Check sheet for the modelled part. Datum: model origin and axes. Units: mm. A direction names the side the tool comes from. Round coordinates to 2 decimals unless told otherwise and drop trailing zeros. Loops run counter-clockwise (first coordinate to the right, second up) from the corner with the lowest first, then second, coordinate; pieces in that order, holes last. Notation, with made-up numbers: (65.5, 0.25) - (118.5, 0.25) arc R18 cw to (118.5, 33.25) - close; hole circle Ø9 at (87.5, -2). An arc over 180 degrees is marked (long way). Put each result on its own line as item: value. Start each with the question number.
Item 1: Gauge pin test, flat ends, axial feed: pin 1 Ø2.5 at (x, z) = (75, -18.75) entering from +Y; pin 2 Ø1 at (x, y) = (-58, 1) entering from -Z. Record the tip position at first contact, or that the pin passes through.
Item 2: Section check B-B, the plane z = 48. Record the cut outline in (x, y), and give its area (3 significant figures).
Item 3: Material ranges on line 1 along X through (y, z) = (2.55, -18.75); line 2 along Z through (x, y) = (60, 1.9); line 3 along X through (y, z) = (1.1, 41), recorded low to high.
Item 4: Section check C-C, the plane x = 47.5. Record the cut outline in (y, z).
Item 5: Section check A-A, the plane y = 1.55. Give the number of separate pieces and of enclosed holes in the cut face, and give its area (3 significant figures).
Item 6: Tool access check on faces 1 (the flat face through (68.25, 2, 54)), 2 (the flat face through (-53, 2, -35.75)), 3 (the flat face through (53, 2, -35.75)), 4 (the flat face through (-68.25, 2, 54)), 5 (the flat face through (1, 2, 72.25)). Record the directions out of +Z, -Z, +X, -X, +Y, -Y that give a thin tool (end or side, any length) a straight path to the whole face; none if there is none.
from build123d import *

# Parameters (mm, degrees)
SKETCH1_R           = 1.5025
BOSS_EXTRUDE1_DEPTH = 3.25


with BuildPart() as part:
    # Sketch1 → Boss-Extrude1 (new body)
    with BuildSketch(Plane(origin=(0, 0, 0), x_dir=(1, 0, 0), z_dir=(0, 1, 0))):
        Polygon((-11, 56.036176716), (11, 56.036176716), (26, 35.75), (80, 35.75), (80, -35.75), (68.25, -35.75), (68.25, -72.25), (-68.25, -72.25), (-68.25, -35.75), (-80, -35.75), (-80, 35.75), (-26, 35.75), align=None)
        with Locations((-10, 33.75)):
            Circle(SKETCH1_R, mode=Mode.SUBTRACT)
        with Locations((10, 33.75)):
            Circle(SKETCH1_R, mode=Mode.SUBTRACT)
        with Locations((-10, 53.75)):
            Circle(SKETCH1_R, mode=Mode.SUBTRACT)
        with Locations((10, 53.75)):
            Circle(SKETCH1_R, mode=Mode.SUBTRACT)
        with Locations((-25, 23.75)):
            Circle(SKETCH1_R, mode=Mode.SUBTRACT)
        with Locations((25, 23.75)):
            Circle(SKETCH1_R, mode=Mode.SUBTRACT)
        with Locations((-60, 18.75)):
            Circle(SKETCH1_R, mode=Mode.SUBTRACT)
        with Locations((60, 18.75)):
            Circle(SKETCH1_R, mode=Mode.SUBTRACT)
        with Locations((75, 18.75)):
            Circle(SKETCH1_R, mode=Mode.SUBTRACT)
        with Locations((-60, -16.25)):
            Circle(SKETCH1_R, mode=Mode.SUBTRACT)
        with Locations((60, -16.25)):
            Circle(SKETCH1_R, mode=Mode.SUBTRACT)
        with Locations((75, -16.25)):
            Circle(SKETCH1_R, mode=Mode.SUBTRACT)
        with Locations((-25, -41.25)):
            Circle(SKETCH1_R, mode=Mode.SUBTRACT)
        with Locations((25, -41.25)):
            Circle(SKETCH1_R, mode=Mode.SUBTRACT)
        with Locations((-65, -66.25)):
            Circle(SKETCH1_R, mode=Mode.SUBTRACT)
        with Locations((-20, -66.25)):
            Circle(SKETCH1_R, mode=Mode.SUBTRACT)
        with Locations((20, -66.25)):
            Circle(SKETCH1_R, mode=Mode.SUBTRACT)
        with Locations((65, -66.25)):
            Circle(SKETCH1_R, mode=Mode.SUBTRACT)
        with Locations((-75, 18.75)):
            Circle(SKETCH1_R, mode=Mode.SUBTRACT)
        with Locations((-75, -16.25)):
            Circle(SKETCH1_R, mode=Mode.SUBTRACT)
    extrude(amount=BOSS_EXTRUDE1_DEPTH)


solid = part.part
Check result:
1. pin 1: through
1. pin 2: z = -35.75
2. outline: (-68.25, 0) - (68.25, 0) - (68.25, 3.25) - (-68.25, 3.25) - close
2. area: 444 mm²
3. line 1: -80 to -76.5, -73.5 to -61.5, -58.5 to 58.5, 61.5 to 73.5, 76.5 to 80
3. line 2: -35.75 to -20.25, -17.25 to 14.75, 17.75 to 72.25
3. line 3: -68.25 to -26.48, -23.52 to 23.52, 26.48 to 68.25
4. outline: (0, -35.75) - (3.25, -35.75) - (3.25, 72.25) - (0, 72.25) - close
5. separate pieces: 1
5. enclosed holes: 20
5. area: 17,000 mm²
6. face 1: +Z, +X, +Y, -Y
6. face 2: -Z, -X, +Y, -Y
6. face 3: -Z, +X, +Y, -Y
6. face 4: +Z, -X, +Y, -Y
6. face 5: +Z, +X, -X, +Y, -Y
